Could you check a few things on this drawing? It's one solid part, dimensions in mm from its lowest x, y, z. A direction names the side the tool comes from. Give positions to 0.01 mm unless a question says otherwise; leave off trailing zeros. Loops run counter-clockwise (first coordinate to the right, second up) from the corner with the lowest first, then second, coordinate; pieces in that order, holes last. Notation, with made-up numbers: M 3.5,0.5 L 33.5,0.5 A18 ccw 33.5,22.5 Z; hole C 85,5 d6. An arc over 180 degrees is marked long. Return JSON: item names as keys, results as strings. Group by question number.
1. Please list where these lines run through material, in increasing order: line 1 (Y direction, x = 34, z = 27.5); line 2 (Y direction, x = 38.5, z = 5); line 3 (Z direction, x = 10, y = 19).
2. For pin 1 (6 mm diameter, centred on y = 30.5, z = 18, fed in from +X); pin 2 (2 mm diameter, centred on x = 25.5, y = 25.5, fed in from -Z); pin 3 (1.5 mm diameter, centred on x = 6.5, y = 15.5, fed in from -Z), each with a flat end and sliding along its axis, tell me the tip position at first contact or that it passes through.
3. If we section it at B-B (x = 20): Write out the boundary of the cut face in (y, z), plus the area to 3 significant figures.
4. For the marked faces 5, 6 and 7, which set-ups out of +Z, -Z, +X, -X, +Y, -Y let a thin tool reach every point of the face, with its end or its side?
5. If we section it at C-C (y = 10): Write out the boundary of the cut face in (x, z).
6. If we section it at A-A (z = 21.5): Write out the boundary of the cut face in (x, y).
7. If we mould it in two halves opening along Y, with no side actions, what happens to the marked faces 1, 2, 3 and 4? For each: +Y half, -Y half, draft (parallel to the pull), parting line (faces both ways), or undercut.
8. If we section it at D-D (y = 33.5): Write out the boundary of the cut face in (x, z).
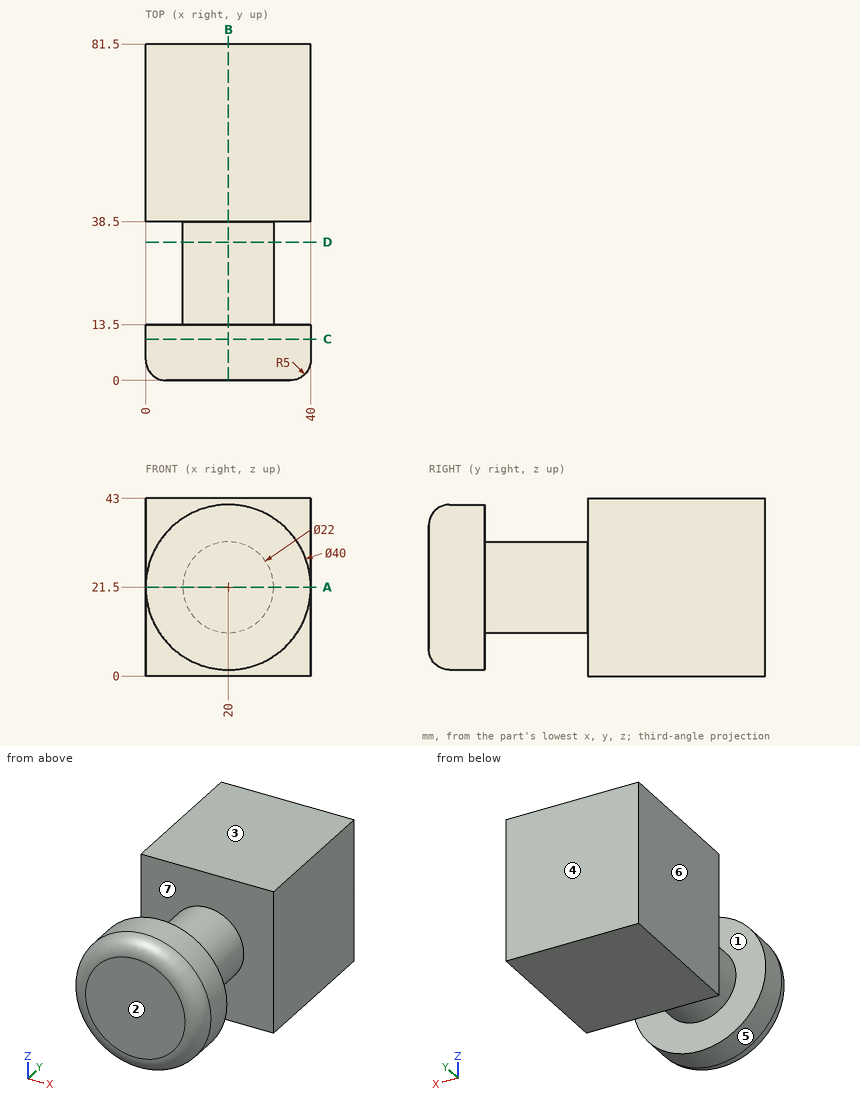
Answer:
{
 "1": {"line 1": "y = 0.01 to 13.5, 38.5 to 81.5", "line 2": "y = 38.5 to 81.5", "line 3": "z = 16.92 to 26.08"},
 "2": {"pin 1": "stops at x = 30.99", "pin 2": "stops at z = 11.46", "pin 3": "passes through"},
 "3": {"outline": "M 0,6.5 A5 ccw 5,1.5 L 13.5,1.5 L 13.5,10.5 L 38.5,10.5 L 38.5,0 L 81.5,0 L 81.5,43 L 38.5,43 L 38.5,32.5 L 13.5,32.5 L 13.5,41.5 L 5,41.5 A5 ccw 0,36.5 Z", "area": "2,930 mm²"},
 "4": {"face 5": "-Y", "face 6": "+Z, -Z, -X, +Y, -Y", "face 7": "none"},
 "5": {"outline": "C 20,21.5 d40"},
 "6": {"outline": "M 0,5 A5 ccw 5,0 L 35,0 A5 ccw 40,5 L 40,13.5 L 31,13.5 L 31,38.5 L 40,38.5 L 40,81.5 L 0,81.5 L 0,38.5 L 9,38.5 L 9,13.5 L 0,13.5 Z"},
 "7": {"face 1": "undercut", "face 2": "-Y half", "face 3": "draft", "face 4": "+Y half"},
 "8": {"outline": "C 20,21.5 d22"}
}
